from build123d import *

# Parameters (mm, degrees)
BOSS_EXTRUDE5_DEPTH = 10
SKETCH3_W           = 5.374011538
SKETCH3_H           = 5.374011538
CUT_EXTRUDE2_DEPTH  = 29.722813389


with BuildPart() as part:
    # Sketch5 → Boss-Extrude5 (new body)
    with BuildSketch(Plane.XY):
        with BuildLine():
            Line((0, 0), (-25, 0))
            add(Edge.make_bspline(
                [(0, 10), (-25, 10), (-25, 0)],
                knots=[4.71238898, 4.71238898, 4.71238898, 6.283185307, 6.283185307, 6.283185307], degree=2, weights=[1, 0.707106781, 1]))
            ThreePointArc((0, 10), (7.071067812, 7.071067812), (10, 0))
            Line((10, 0), (0, 0))
        make_face()
    extrude(amount=-BOSS_EXTRUDE5_DEPTH)

    # Mirror2: part across plane


with BuildPart() as part_1:
    add(part.part)
    add(part.part.mirror(Plane(origin=(0, 0, -10), x_dir=(0, 0, 1), z_dir=(0, -1, 0))))

    # Sketch3 → Cut-Extrude2 (cut, through all)
    with BuildSketch(Plane.XY):
        Rectangle(SKETCH3_W, SKETCH3_H)
    extrude(amount=-CUT_EXTRUDE2_DEPTH, mode=Mode.SUBTRACT)


solid = part_1.part
Design review of the part built by this model. Coordinates are the model's own, in mm. A direction names the side the tool comes from. Round coordinates to 2 decimals unless told otherwise and drop trailing zeros. Order: outer loops, then holes, each group sorted by start corner. A loop starts at its lowest first (then second) coordinate and runs counter-clockwise, first axis right, second up.
1) Clearance check with flat-ended pins moving along their axes: pin 1 Ø3 at (x, z) = (6, -2.5) entering from -Y; pin 2 Ø4 at (y, z) = (-7.5, -5) entering from -X; pin 3 Ø3 at (x, z) = (-5.5, -3) entering from -Y. State where each tip first meets the part, or that it passes through.
The answers:
pin 1: stops at y = -8.93
pin 2: stops at x = -20.88
pin 3: stops at y = -9.87
2) Consider section A-A (x = 7). State the section outline as (y, z) points, plus the area to 3 significant figures.
The answers:
outline: (-7.14, -10) - (7.14, -10) - (7.14, 0) - (-7.14, 0) - close
area: 143 mm2
3) For L1, parallel to X at y = 0, z = -2.5; L2, parallel to Y at x = -1, z = -6.75; L3, parallel to X at y = 0.75, z = -7.5, list the stretches that pass through material, from the lowest coordinate up.
The answers:
L1: x = -25 to -2.69, 2.69 to 10
L2: y = -9.99 to -2.69, 2.69 to 9.99
L3: x = -24.93 to -2.69, 2.69 to 9.97
4) Draft analysis for pull direction X (two halves, no side actions). For faces 1 (the flat face through (-2.687, 0, -5)), 2 (the flat face through (0, 2.687, -5)), 3 (the flat face through (-8, 0, 0)), state which applies: released by +X, released by -X, zero draft, split by the parting line, or undercut.
The answers:
face 1: undercut
face 2: undercut
face 3: zero draft
5) Machinability: for faces 4 (the flat face through (-8, 0, -10)), 5 (the flat face through (2.687, 0, -5)), which of the approach directions +Z, -Z, +X, -X, +Y, -Y give a long, thin tool a straight path to every point of the face, cutting with its end or side? Answer none if there is none.
The answers:
face 4: -Z, +X, -X, +Y, -Y
face 5: +Z, -Z
